Part model, mm, in its own coordinate system. Face numbers are marked on the shaded views. A direction names the side the tool comes from. Round coordinates to 2 decimals unless told otherwise and drop trailing zeros. Write each loop counter-clockwise with the first axis right and the second up, starting at its lowest first coordinate (ties: lowest second). Pieces come first, ordered by that corner, then holes.
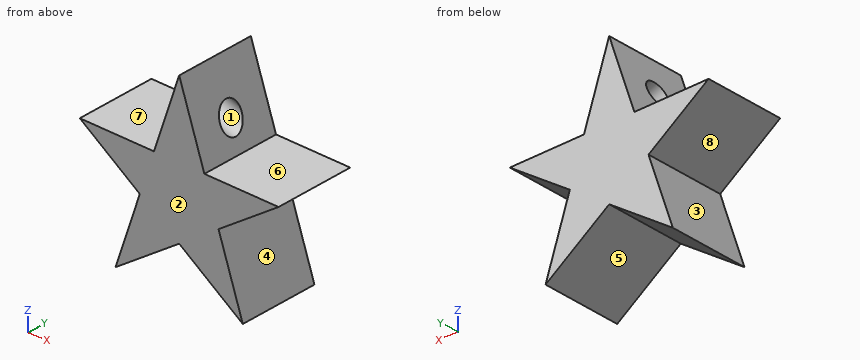
from build123d import *

# Parameters (mm, degrees)
F1_DEPTH = 15.24
F3_R     = 2.312647279
F4_DEPTH = 10.6426


with BuildPart() as f1:
    # F0 (on Front) → F1 (new body)
    with BuildSketch(Plane.XZ):
        Polygon((-7.3665321659, 21.7996356664), (-12.1971740292, 36.0948603779), (-17.0278158926, 21.7996356664), align=None)
        Polygon((-7.3665321659, 21.7996356664), (-17.0278158926, 21.7996356664), (-19.7405148125, 13.7719984015), (-12.1971740292, 8.5093759118), (-4.6538332459, 13.7719984015), align=None)
        Polygon((-19.7405148125, 13.7719984015), (-17.0278158926, 21.7996356664), (-31.2471740292, 21.7996356664), align=None)
        Polygon((6.8528259708, 21.7996356664), (-7.3665321659, 21.7996356664), (-4.6538332459, 13.7719984015), align=None)
        Polygon((-12.1971740292, 8.5093759118), (-19.7405148125, 13.7719984015), (-24.3943480584, 0), align=None)
        Polygon((0, 0), (-4.6538332459, 13.7719984015), (-12.1971740292, 8.5093759118), align=None)
    extrude(amount=F1_DEPTH)

    # F3 (on face) → F4 (cut)
    with BuildSketch(Plane(origin=(-21.8942461856, 0, 7.3985029494), x_dir=(0, -1, 0), z_dir=(-0.9473716635, 0, 0.3201358013))):
        with Locations((7.62, 22.7458197282)):
            Circle(F3_R)
    extrude(amount=-F4_DEPTH, mode=Mode.SUBTRACT)


solid = f1.part
Q1. Wall check: line 1 (Y direction, x = -8.5, z = 25); line 2 (X direction, y = -9.75, z = 6); line 3 (Y direction, x = -11.5, z = 29.5). Give the ranges that are in metal, low to high.
Q2. Two-plate mould, pull along Y, no slides. Class the marked faces 1, 2 and 3: released by +Y, released by -Y, zero draft, split by the parting line, or undercut.
Q3. Saw through at B-B, the plane x = -21. Write the cut outline in (y, z), and give its area (3 significant figures).
Q4. Saw through at C-C, the plane z = 5. Write the cut outline in (x, y).
Q5. Drop flat-ended pins along their axis: P1, Ø7, axis at x = 1.5, y = -5.5, coming from the +Z side; P2, Ø3, axis at x = -22.5, y = -3, coming from the -Z side; P3, Ø3, axis at y = -13, z = 23, coming from the -X side. Give the stop position or say it passes through.
Q6. Tool access for the marked faces 4, 5, 6, 7 and 8: list every direction of +Z, -Z, +X, -X, +Y, -Y with a clear straight run to the whole face (end or side of a thin tool).
Q7. Saw through at A-A, the plane y = -5.75. Write the cut outline in (x, z).
Q8. Saw through at D-D, the plane z = 14.5. Write the cut outline in (x, y).
Computed:
1. line 1: y = -15.24 to -9.09, -6.15 to 0
1. line 2: x = -22.37 to -15.79, -8.6 to -2.03
1. line 3: y = -15.24 to -9.36, -5.88 to 0
2. face 1: undercut
2. face 2: released by -Y
2. face 3: zero draft
3. outline: (-15.24, 2.37) - (0, 2.37) - (0, 10.04) - (-15.24, 10.04) - close; (-15.24, 14.65) - (0, 14.65) - (0, 21.8) - (-15.24, 21.8) - close
3. area: 226 mm2
4. outline: (-22.7, -15.24) - (-17.23, -15.24) - (-17.23, 0) - (-22.7, 0) - close; (-7.17, -15.24) - (-1.69, -15.24) - (-1.69, 0) - (-7.17, 0) - close
5. P1: stops at z = 21.8
5. P2: stops at z = 0.28
5. P3: stops at x = -31.25
6. face 4: +X, +Y, -Y
6. face 5: -Z, +Y, -Y
6. face 6: +Z, +X, +Y, -Y
6. face 7: +Z, -X, +Y, -Y
6. face 8: -X, +Y, -Y
7. outline: (-31.25, 21.8) - (-19.74, 13.77) - (-24.39, 0) - (-12.2, 8.51) - (0, 0) - (-4.65, 13.77) - (6.85, 21.8) - (-7.37, 21.8) - (-8.61, 25.48) - (-15.05, 27.66) - (-17.03, 21.8) - close; (-14.18, 30.24) - (-9.71, 28.73) - (-12.2, 36.09) - close
8. outline: (-20.78, -15.24) - (-3.61, -15.24) - (-3.61, 0) - (-20.78, 0) - close
